Geometry: final body of the model. Coordinates: model frame, mm. Face numbers are marked on the shaded views. A direction names the side the tool comes from. Round coordinates to 2 decimals unless told otherwise and drop trailing zeros. Write each loop counter-clockwise with the first axis right and the second up, starting at its lowest first coordinate (ties: lowest second). Pieces come first, ordered by that corner, then holes. Notation, with made-up numbers: M -4.75,-16.5 L 40.25,-16.5 A26 ccw 40.25,4.5 Z; hole C 69,56.25 d6. An arc over 180 degrees is marked long. Use one line per item in the form item = value. Start each with the question number.
Item 1: Pull-direction query (Y, two-part tool) for the marked faces 4, 5 and 6; classes: pulls with the +Y half, pulls with the -Y half, needs draft (parallel to the pull), parting line crosses it, or undercut.
Item 2: Pin query (flat end, axial travel): pin 1 Ø3 at (x, y) = (-15, 8) entering from -Z; pin 2 Ø5 at (x, z) = (-4.5, 24.5) entering from -Y; pin 3 Ø5.5 at (y, z) = (-7.5, 19) entering from +X; pin 4 Ø9.5 at (x, z) = (7, 10) entering from -Y. Return the tip coordinate at first contact, or that it passes through.
Item 3: Reachability of the marked faces 1, 2 and 3 from +Z, -Z, +X, -X, +Y, -Y: full face, straight path, thin tool, end or side. Return the list, or none.
Item 4: Section query A-A (x = 11). Return loops of the section in (y, z), and give its area (3 significant figures).
Item 5: Ray query, probe 1 along X at (y, z) = (1.5, 9.5); probe 2 along Y at (x, z) = (-14.5, 13); probe 3 along Z at (x, y) = (-15, 7). Return the intervals inside material, ascending.
Item 6: Section query C-C (y = -10). Return loops of the section in (x, z), and give its area (3 significant figures).
Item 7: Section query B-B (z = 2.75). Return loops of the section in (x, y), and give its area (3 significant figures).
from build123d import *

# Parameters (mm, degrees)
F1_DEPTH  = 28
F3_R      = 5.25
F4_DEPTH  = 25
F6_DEPTH  = 3
F7_R      = 4
F8_DEPTH  = 6.5
F9_W      = 2
F9_H      = 3
F9_W_2    = 3
F9_H_2    = 2
F10_DEPTH = 28.001
F2_R      = 5.25
F11_DEPTH = 25
F12_R     = 1
F13_R     = 2


with BuildPart() as f1:
    # F0 (on Top) → F1 (new body)
    with BuildSketch(Plane.XY):
        Polygon((-19.75, 3.25), (-19.75, -19.75), (-17.75, -19.75), (-17.75, 2.421573), (-2.421573, 17.75), (19.75, 17.75), (19.75, 19.75), (-3.25, 19.75), (-7.492641, 19.75), (-19.75, 7.492641), align=None)
    extrude(amount=F1_DEPTH)

    # F3 (on face) → F4 (cut)
    with BuildSketch(Plane.XZ.offset(-17.75)):
        with Locations((6.664214, 14)):
            Circle(F3_R)
    extrude(amount=-F4_DEPTH, mode=Mode.SUBTRACT)

    # F5 (on face) → F6 (cut)
    with BuildSketch(Plane(origin=(-10.085786, 10.085786, 0), x_dir=(0.707107, 0.707107, 0), z_dir=(0.707107, -0.707107, 0))):
        Polygon((-3.897114, 7.25), (3.897114, 7.25), (7.794229, 14), (3.897114, 20.75), (-3.897114, 20.75), (-7.794229, 14), align=None)
    extrude(amount=-F6_DEPTH, mode=Mode.SUBTRACT)

    # F7 (on face) → F8 (join)
    with BuildSketch(Plane(origin=(-12.207107, 12.207107, 0), x_dir=(0.707107, 0.707107, 0), z_dir=(0.707107, -0.707107, 0))):
        Polygon((3.752777, 20.5), (-3.752777, 20.5), (-7.505553, 14), (-3.752777, 7.5), (3.752777, 7.5), (7.505553, 14), align=None)
        with Locations((0, 14)):
            Circle(F7_R, mode=Mode.SUBTRACT)
    extrude(amount=F8_DEPTH)

    # F9 (on face) → F10 (cut, through all)
    with BuildSketch(Plane.XY.offset(28)):
        with Locations((-18.75, -18.25)):
            Rectangle(F9_W, F9_H)
        with Locations((18.25, 18.75)):
            Rectangle(F9_W_2, F9_H_2)
    extrude(amount=-F10_DEPTH, mode=Mode.SUBTRACT)

    # F2 (on face) → F11 (cut)
    with BuildSketch(Plane.YZ.offset(-17.75)):
        with Locations((-6.664214, 14)):
            Circle(F2_R)
    extrude(amount=-F11_DEPTH, mode=Mode.SUBTRACT)

    # F12
    f12_edges = [f1.edges().sort_by_distance(p)[0] for p in [
        (-17.75, 2.421573, 14),
        (-2.421573, 17.75, 14),
        (16.75, 18.75, 28),
        (16.75, 18.75, 0),
        (-18.75, -16.75, 28),
        (-18.75, -16.75, 0),
    ]]
    fillet(f12_edges, radius=F12_R)

    # F13
    f13_edges = [f1.edges().sort_by_distance(p)[0] for p in [
        (-19.75, 7.492641, 14),
        (-7.492641, 19.75, 14),
    ]]
    fillet(f13_edges, radius=F13_R)


solid = f1.part
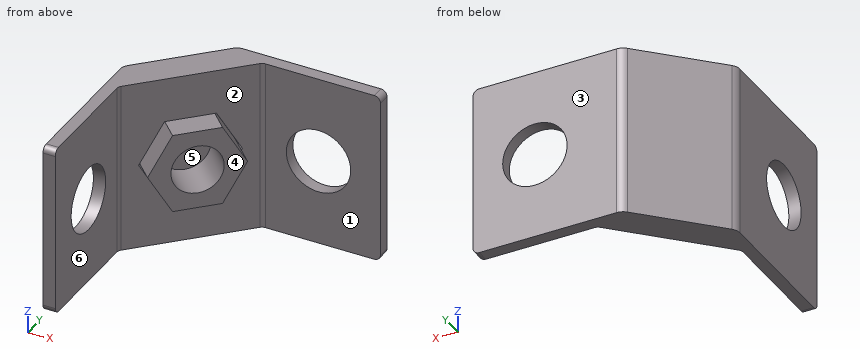
Working result:
q1.face_4 = pulls with the -Y half
q1.face_5 = undercut
q1.face_6 = needs draft
q2.pin_1 = 0
q2.pin_2 = 13.17
q2.pin_3 = -17.75
q2.pin_4 = 17.75
q3.face_1 = +Z, -Z, +X, -Y
q3.face_2 = none
q3.face_3 = +Z, -Z, +X, -X, +Y
q4.outline = M 17.75,0 L 19.75,0 L 19.75,11.04 L 17.75,11.04 Z; M 17.75,16.96 L 19.75,16.96 L 19.75,28 L 17.75,28 Z
q4.area = 44.2 mm²
q5.probe_1 = -19.75 to -17.75
q5.probe_2 = 4.7 to 9.02, 9.91 to 12.74
q5.probe_3 = 0 to 10.3, 10.8 to 17.2, 17.7 to 28
q6.outline = M -19.75,0 L -17.75,0 L -17.75,9.95 L -19.75,9.95 Z; M -19.75,18.05 L -17.75,18.05 L -17.75,28 L -19.75,28 Z
q6.area = 39.8 mm²
q7.outline = M -19.75,-16.75 L -17.75,-16.75 L -17.75,2.01 A1 cw -17.46,2.71 L -2.71,17.46 A1 cw -2.01,17.75 L 16.75,17.75 L 16.75,19.75 L -6.66,19.75 A2 ccw -8.08,19.16 L -19.16,8.08 A2 ccw -19.75,6.66 Z
q7.area = 184 mm²
